Design review of the part built by this model. Coordinates are the model's own, in mm. Face numbers are marked on the shaded views. Round coordinates to 2 decimals unless told otherwise and drop trailing zeros. Order: outer loops, then holes, each group sorted by start corner. A loop starts at its lowest first (then second) coordinate and runs counter-clockwise, first axis right, second up. Notation, with made-up numbers: (61.25, 17.5) - (116.25, 17.5) arc R13 ccw to (116.25, 41.5) - close; hole circle Ø7 at (28, 5.25). An arc over 180 degrees is marked (long way). Write item = value, one per line.
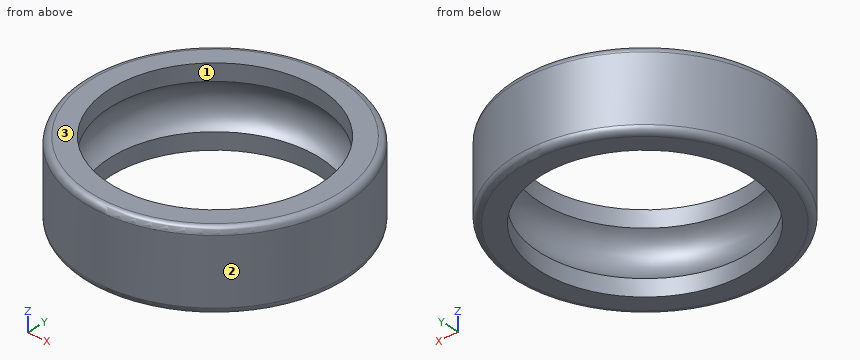
from build123d import *

# Parameters (mm, degrees)
SKETCH1_R           = 10
SKETCH1_R_2         = 8
BOSS_EXTRUDE1_DEPTH = 3
SKETCH2_R           = 2
FILLET1_R           = 0.5


with BuildPart() as part:
    # Sketch1 → Boss-Extrude1 (new, symmetric)
    with BuildSketch(Plane.XY):
        Circle(SKETCH1_R)
        Circle(SKETCH1_R_2, mode=Mode.SUBTRACT)
    extrude(amount=BOSS_EXTRUDE1_DEPTH, both=True)

    # Sketch2 → Cut-Revolve1 (revolve, cut)
    with BuildSketch(Plane(origin=(0, 0, 0), x_dir=(1, 0, 0), z_dir=(0, 1, 0))):
        with Locations((-7, 0)):
            Circle(SKETCH2_R)
    revolve(axis=Axis((0, 0, -1.800319694), (0, 0, 1)), mode=Mode.SUBTRACT)

    # Fillet1
    fillet1_edges = [part.edges().sort_by_distance(p)[0] for p in [
        (-10, 0, -3),
        (-10, 0, 3),
    ]]
    fillet(fillet1_edges, radius=FILLET1_R)


solid = part.part
Item 1: The part is to be moulded in two halves that separate along Y. For the marked faces 1, 2 and 3, say which applies: +Y half, -Y half, draft (parallel to the pull), parting line (faces both ways), or undercut.
Data:
face_1 = undercut
face_2 = parting line
face_3 = draft
Item 2: Insertion check: P1, Ø1, axis at y = 7.5, z = 0.5, coming from the -X side; P2, Ø1.5, axis at x = -4.5, z = 0, coming from the +Y side; P3, Ø1, axis at y = -6, z = -1, coming from the +X side. Each pin has a flat end and moves straight along its axis. Give the tip position at first contact, or say it passes through.
Data:
P1 = -7.14
P2 = 9.27
P3 = 8.35
Item 3: For line 1 along Y through (x, z) = (0, -2.45); line 2 along Y through (x, z) = (-4.75, 2.25); line 3 along X through (y, z) = (0.5, 0.25), list the stretches that pass through material, from the lowest coordinate up. Write a range as [from, to].
Data:
line_1 = [-10, -8], [8, 10]
line_2 = [-8.8, -6.44], [6.44, 8.8]
line_3 = [-9.99, -8.97], [8.97, 9.99]
Item 4: Take a section at A-A, the plane x = 0. State the section outline as (y, z) points, and give its area (3 significant figures).
Data:
outline = (-10, -2.5) arc R0.5 ccw to (-9.5, -3) - (-8, -3) - (-8, -1.73) arc R2 cw to (-8, 1.73) - (-8, 3) - (-9.5, 3) arc R0.5 ccw to (-10, 2.5) - close; (8, -3) - (9.5, -3) arc R0.5 ccw to (10, -2.5) - (10, 2.5) arc R0.5 ccw to (9.5, 3) - (8, 3) - (8, 1.73) arc R2 cw to (8, -1.73) - close
area = 18.9 mm2
